```python
from build123d import *

# Parameters (mm, degrees)
EXTRUDE_2_DEPTH     = 60
CUT_EXTRUDE_2_DEPTH = 189.939286944
SKETCH_7_R          = 25
CUT_EXTRUDE_4_DEPTH = 20
SKETCH_8_R          = 25
CUT_EXTRUDE_5_DEPTH = 20


with BuildPart() as part:
    # 草图1 → 凸台-拉伸2 (new body)
    with BuildSketch(Plane.XY):
        Polygon((-161.784091828, 76.967277349), (-161.784091828, 16.967277349), (-127.826106531, -63.032722651), (-27.826106531, -63.032722651), (6.131878766, 16.967277349), (6.131878766, 76.967277349), align=None)
    extrude(amount=EXTRUDE_2_DEPTH)

    # 草图5 → 切除-拉伸2 (cut, through all)
    with BuildSketch(Plane.XY.offset(60)):
        Polygon((-141.784091828, 76.967277349), (-141.784091828, 16.967277349), (-112.836441026, -51.229114277), (-42.815772036, -51.229114277), (-13.868121234, 16.967277349), (-13.868121234, 76.967277349), align=None)
    extrude(amount=-CUT_EXTRUDE_2_DEPTH, mode=Mode.SUBTRACT)

    # 草图7 → 切除-拉伸4 (cut)
    with BuildSketch(Plane.ZY.offset(161.784091828)):
        with Locations(Location((30, 46.967277349, 0), (0, 0, 270))):
            Circle(SKETCH_7_R)
    extrude(amount=-CUT_EXTRUDE_4_DEPTH, mode=Mode.SUBTRACT)

    # 草图8 → 切除-拉伸5 (cut)
    with BuildSketch(Plane(origin=(0, -51.229114277, 0), x_dir=(1, 0, 0), z_dir=(0, 1, 0))):
        with Locations(Location((-77.815772036, -30, 0), (0, 0, 270))):
            Circle(SKETCH_8_R)
    extrude(amount=-CUT_EXTRUDE_5_DEPTH, mode=Mode.SUBTRACT)


solid = part.part
```
Here's how the part is built. I have some questions about the finished solid (model axes, mm). A direction names the side the tool comes from. Round coordinates to 2 decimals unless told otherwise and drop trailing zeros. Order: outer loops, then holes, each group sorted by start corner. A loop starts at its lowest first (then second) coordinate and runs counter-clockwise, first axis right, second up. Notation, with made-up numbers: M 58,-23 L 75,-23 A11 cw 75,-11 Z; hole C -36,-7.75 d11. An arc over 180 degrees is marked long. Answer as CSV lines item,"result".
Item 1: Imagine slicing it at A-A on z = 30. List the corners of the cut face in (x, y) for me, and give its area (3 significant figures).
From the geometry:
outline,"M -161.78,16.97 L -127.83,-63.03 L -102.82,-63.03 L -102.82,-51.23 L -112.84,-51.23 L -141.78,16.97 L -141.78,21.97 L -161.78,21.97 Z; M -161.78,71.97 L -141.78,71.97 L -141.78,76.97 L -161.78,76.97 Z; M -52.82,-63.03 L -27.83,-63.03 L 6.13,16.97 L 6.13,76.97 L -13.87,76.97 L -13.87,16.97 L -42.82,-51.23 L -52.82,-51.23 Z"
area,"4,780 mm2"
Item 2: Which directions (+Z, -Z, +X, -X, +Y, -Y) give clear straight access to the entire face, cutting with the end or side of a thin tool? Please do faces 1 (the flat face through (-28.545, -17.608, 30.42)), 2 (the flat face through (-161.784, 21, 30)).
From the geometry:
face 1,"+Z, -Z, +Y"
face 2,"+Z, -Z, -X, +Y, -Y"
Item 3: Imagine slicing it at B-B on x = -66. List the corners of the cut face in (y, z) for me, and give its area (3 significant figures).
From the geometry:
outline,"M -63.03,0 L -51.23,0 L -51.23,7.97 L -63.03,7.97 Z; M -63.03,52.03 L -51.23,52.03 L -51.23,60 L -63.03,60 Z"
area,"188 mm2"
Item 4: Please list where these lines run through material, in increasing order: L1, parallel to X at y = 68, z = 9.5; L2, parallel to X at y = 61, z = 32; L3, parallel to X at y = -55, z = 30. Write a range as [from, to].
From the geometry:
L1,"[-161.78, -141.78], [-13.87, 6.13]"
L2,"[-13.87, 6.13]"
L3,"[-131.24, -102.82], [-52.82, -24.42]"
Item 5: Imagine slicing it at C-C on y = 68. List the corners of the cut face in (x, z) for me, and give its area (3 significant figures).
From the geometry:
outline,"M -161.78,0 L -141.78,0 L -141.78,16.49 L -161.78,16.49 Z; M -161.78,43.51 L -141.78,43.51 L -141.78,60 L -161.78,60 Z; M -13.87,0 L 6.13,0 L 6.13,60 L -13.87,60 Z"
area,"1,860 mm2"
Item 6: We'd pull the mould along Y, two halves only. Please class faces 3 (the cylindrical face through (-60.92, -57.048, 11.574)), 4 (the cylindrical face through (-151.92, 35.43, 7.82)), 5 (the flat face through (-94, -51.229, 50)): +Y half, -Y half, draft (parallel to the pull), parting line (faces both ways), or undercut.
From the geometry:
face 3,"draft"
face 4,"undercut"
face 5,"+Y half"
Item 7: For pin 1 (10 mm diameter, centred on x = -22, z = 46.5, fed in from -Y); pin 2 (8 mm diameter, centred on y = -2.5, z = 35.5, fed in from -X); pin 3 (18 mm diameter, centred on y = 42, z = 40, fed in from -X); pin 4 (1.5 mm diameter, centred on x = -100, z = 33.5, fed in from +Y), each with a flat end and sliding along its axis, tell me the tip position at first contact or that it passes through.
From the geometry:
pin 1,"y = -61.09"
pin 2,"x = -155.22"
pin 3,"x = -13.87"
pin 4,"through"
Item 8: Imagine slicing it at D-D on y = -33. List the corners of the cut face in (x, z) for me, and give its area (3 significant figures).
From the geometry:
outline,"M -140.57,0 L -120.57,0 L -120.57,60 L -140.57,60 Z; M -35.08,0 L -15.08,0 L -15.08,60 L -35.08,60 Z"
area,"2,400 mm2"
